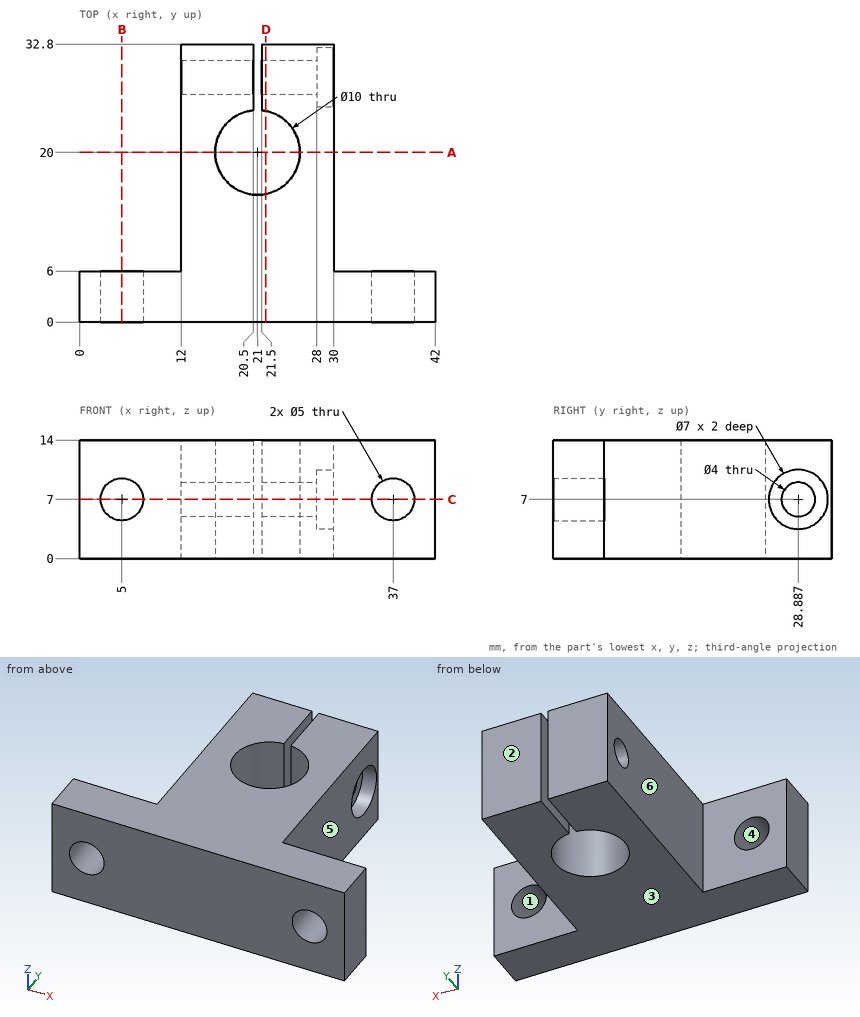
Source: three-view drawing plus pictorial views. Frame: mm from the lowest corner of the part. A direction names the side the tool comes from. Give positions to 0.01 mm unless a question says otherwise; leave off trailing zeros. Order: outer loops, then holes, each group sorted by start corner. A loop starts at its lowest first (then second) coordinate and runs counter-clockwise, first axis right, second up.
1. Pin query (flat end, axial travel): pin 1 (2 mm diameter, centred on y = 12, z = 3, fed in from +X); pin 2 (5 mm diameter, centred on y = 23.5, z = 7, fed in from -X); pin 3 (8 mm diameter, centred on x = 34, y = 9, fed in from -Z); pin 4 (2.5 mm diameter, centred on y = 28.89, z = 7, fed in from -X). Return the tip coordinate at first contact, or that it passes through.
Derived:
pin 1: stops at x = 30
pin 2: stops at x = 12
pin 3: stops at z = 0
pin 4: passes through
2. Reachability of the marked faces 4, 5 and 6 from +Z, -Z, +X, -X, +Y, -Y: full face, straight path, thin tool, end or side. Return the list, or none.
Derived:
face 4: +Y, -Y
face 5: +Z, -Z, +X, +Y
face 6: +Z, -Z, -X, +Y
3. Mould query, pull axis Z, two halves, no side actions, for the marked faces 1, 2 and 3. Classes: released by +Z, released by -Z, zero draft, split by the parting line, or undercut.
Derived:
face 1: undercut
face 2: zero draft
face 3: released by -Z
4. Material intervals for L1, parallel to X at y = 3.15, z = 7; L2, parallel to X at y = 30.5, z = 2.25; L3, parallel to X at y = 28, z = 10, sorted ascending.
Derived:
L1: x = 0 to 2.5, 7.5 to 34.5, 39.5 to 42
L2: x = 12 to 20.5, 21.5 to 30
L3: x = 12 to 20.5, 21.5 to 28
5. Section D-D on x = 22. Return the cut outline in (y, z).
Derived:
outline: (0, 0) - (15.1, 0) - (15.1, 14) - (0, 14) - close; (24.9, 0) - (32.8, 0) - (32.8, 14) - (24.9, 14) - close; hole circle Ø4 at (28.89, 7)
6. Section C-C on z = 7. Give the number of separate pieces and of enclosed holes in the cut face, and give its area (3 significant figures).
Derived:
separate pieces: 5
enclosed holes: 0
area: 514 mm2
7. Section B-B on x = 5. Return the cut outline in (y, z).
Derived:
outline: (0, 0) - (6, 0) - (6, 4.5) - (0, 4.5) - close; (0, 9.5) - (6, 9.5) - (6, 14) - (0, 14) - close
8. Section A-A on y = 20. Return the cut outline in (x, z).
Derived:
outline: (12, 0) - (16, 0) - (16, 14) - (12, 14) - close; (26, 0) - (30, 0) - (30, 14) - (26, 14) - close
